```python
from build123d import *

# Parameters (mm, degrees)
STOCK_BOX_1_OUTLINE_W   = 122
STOCK_BOX_1_OUTLINE_H   = 102
STOCK_BOX_1_OUTLINE_W_2 = 118
STOCK_BOX_1_OUTLINE_H_2 = 98
STOCK_BOX_1_DEPTH       = 67
STOCK_BOX_1_2_OUTLINE_W = 118
STOCK_BOX_1_2_OUTLINE_H = 98
STOCK_BOX_1_2_DEPTH     = 2
SKETCH1_W               = 97
SKETCH1_H               = 39.5
CUT_EXTRUDE1_DEPTH      = 10
SKETCH2_W               = 15
SKETCH2_H               = 7.5
CUT_EXTRUDE2_DEPTH      = 10
SKETCH3_W               = 122
SKETCH3_H               = 5
BOSS_EXTRUDE1_DEPTH     = 11
SKETCH5_W               = 122
SKETCH5_H               = 5
BOSS_EXTRUDE2_DEPTH     = 49.5
SKETCH6_W               = 19
SKETCH6_H               = 15
SKETCH6_W_2             = 11
SKETCH6_H_2             = 11
CUT_EXTRUDE3_DEPTH      = 50


# Read off the part's stored shape, not the designer's step: Stock-Box-1
with BuildPart() as part:
    # Stock-Box-1 outline → Stock-Box-1 (new body)
    with BuildSketch(Plane(origin=(0, 0, 0), x_dir=(1, 0, 0), z_dir=(0, 1, 0))):
        with Locations((6.476673428, -22.886409736)):
            Rectangle(STOCK_BOX_1_OUTLINE_W, STOCK_BOX_1_OUTLINE_H)
        with Locations((6.476673428, -22.886409736)):
            Rectangle(STOCK_BOX_1_OUTLINE_W_2, STOCK_BOX_1_OUTLINE_H_2, mode=Mode.SUBTRACT)
    extrude(amount=STOCK_BOX_1_DEPTH)

    # Stock-Box-1 2 outline → Stock-Box-1 2 (add)
    with BuildSketch(Plane(origin=(0, 0, 0), x_dir=(1, 0, 0), z_dir=(0, 1, 0))):
        with Locations((6.476673428, -22.886409736)):
            Rectangle(STOCK_BOX_1_2_OUTLINE_W, STOCK_BOX_1_2_OUTLINE_H)
    extrude(amount=STOCK_BOX_1_2_DEPTH)

    # Sketch1 → Cut-Extrude1 (cut)
    with BuildSketch(Plane.XY.offset(73.886409736)):
        with Locations((6.476673428, 34.25)):
            Rectangle(SKETCH1_W, SKETCH1_H)
    extrude(amount=-CUT_EXTRUDE1_DEPTH, mode=Mode.SUBTRACT)

    # Sketch2 → Cut-Extrude2 (cut)
    with BuildSketch(Plane(origin=(0, 0, -28.113590264), x_dir=(-1, 0, 0), z_dir=(0, 0, -1))):
        with Locations((-22.476673428, 58.25)):
            Rectangle(SKETCH2_W, SKETCH2_H)
        with Locations((29.523326572, 58.25)):
            Rectangle(SKETCH2_W, SKETCH2_H)
    extrude(amount=-CUT_EXTRUDE2_DEPTH, mode=Mode.SUBTRACT)

    # Sketch3 → Boss-Extrude1 (add)
    with BuildSketch(Plane(origin=(0, 0, -28.113590264), x_dir=(-1, 0, 0), z_dir=(0, 0, -1))):
        with Locations((-6.476673428, 52)):
            Rectangle(SKETCH3_W, SKETCH3_H)
    extrude(amount=BOSS_EXTRUDE1_DEPTH)

    # Sketch5 → Boss-Extrude2 (add)
    with BuildSketch(Plane.XZ.offset(-49.5)):
        with Locations((6.476673428, -36.613590264)):
            Rectangle(SKETCH5_W, SKETCH5_H)
    extrude(amount=BOSS_EXTRUDE2_DEPTH)

    # Sketch6 → Cut-Extrude3 (cut)
    with BuildSketch(Plane.ZY.offset(54.523326572)):
        with Locations((-3.613590264, 59.5)):
            Rectangle(SKETCH6_W, SKETCH6_H)
        with Locations((21.386409736, 61.5)):
            Rectangle(SKETCH6_W_2, SKETCH6_H_2)
    extrude(amount=-CUT_EXTRUDE3_DEPTH, mode=Mode.SUBTRACT)


solid = part.part
```
Can you work these out from the model? Positions are in its coordinate system, mm. A direction names the side the tool comes from. Give positions to 0.01 mm unless a question says otherwise; leave off trailing zeros. Order: outer loops, then holes, each group sorted by start corner. A loop starts at its lowest first (then second) coordinate and runs counter-clockwise, first axis right, second up. Notation, with made-up numbers: M 63.25,-12 L 88.25,-12 A32 cw 88.25,27 Z; hole C 11,28.5 d2. An arc over 180 degrees is marked long. Write item = value, one per line. Start each with the question number.
Q1. Will these pins go through, and if not, where does the flat tip stop? pin 1 Ø1 at (x, y) = (-53.5, 61) entering from -Z; pin 2 Ø2 at (x, y) = (-29.5, 57.5) entering from -Z; pin 3 Ø10 at (x, z) = (26, 31) entering from -Y; pin 4 Ø4 at (x, z) = (25.5, -36) entering from +Y.
Q2. We'd pull the mould along X, two halves only. Please class faces 1 (the flat face through (6, 0, 22)), 2 (the flat face through (65.477, 34, 24)), 3 (the flat face through (-54.523, 34, 29)): pulls with the +X half, pulls with the -X half, needs draft (parallel to the pull), parting line crosses it, or undercut.
Q3. Suppose I cut it at D-D (z = 51.5). Write out the boundary of the cut face in (x, y).
Q4. Suppose I cut it at B-B (x = -11.5). Write out the boundary of the cut face in (y, z).
Q5. For faces 4 (the flat face through (6, 12, 71.886)), 5 (the flat face through (67.477, 34, 17)), 6 (the flat face through (6, 25, -34.114)), 7 (the flat face through (6, 61, -28.114)), which set-ups out of +Z, -Z, +X, -X, +Y, -Y let a thin tool reach every point of the face, with its end or its side?
Q6. Suppose I cut it at A-A (x = -31.5). Write out the boundary of the cut face in (y, z), plus the area to 4 significant figures.
Q7. I need wall thicknesses on probe 1 along X at (y, z) = (28.5, 24); probe 2 along Z at (x, y) = (10.5, 16); probe 3 along Z at (x, y) = (-2, 60). Which ranges of each line are inside material? Lowest first, please. Write a range as [from, to].
Q8. Suppose I cut it at C-C (y = 37.5). Write out the boundary of the cut face in (x, z), plus the area to 3 significant figures.
Check result:
q1.pin_1 = -28.11
q1.pin_2 = 71.89
q1.pin_3 = 0
q1.pin_4 = 54.5
q2.face_1 = needs draft
q2.face_2 = undercut
q2.face_3 = pulls with the -X half
q3.outline = M -54.52,0 L 67.48,0 L 67.48,67 L 65.48,67 L 65.48,2 L -52.52,2 L -52.52,67 L -54.52,67 Z
q4.outline = M 0,-39.11 L 54.5,-39.11 L 54.5,-28.11 L 67,-28.11 L 67,-26.11 L 2,-26.11 L 2,71.89 L 14.5,71.89 L 14.5,73.89 L 0,73.89 L 0,-28.11 L 49.5,-28.11 L 49.5,-34.11 L 0,-34.11 Z; M 54,71.89 L 67,71.89 L 67,73.89 L 54,73.89 Z
q5.face_4 = +Y
q5.face_5 = +Z, -Z, +X, +Y, -Y
q5.face_6 = +X, -X, -Y
q5.face_7 = -Z, +X, -X, +Y
q6.outline = M 0,-39.11 L 54.5,-39.11 L 54.5,-26.11 L 2,-26.11 L 2,71.89 L 14.5,71.89 L 14.5,73.89 L 0,73.89 L 0,-28.11 L 49.5,-28.11 L 49.5,-34.11 L 0,-34.11 Z; M 54,71.89 L 67,71.89 L 67,73.89 L 54,73.89 Z; M 62,-28.11 L 67,-28.11 L 67,-26.11 L 62,-26.11 Z
q6.area = 672.5 mm2
q7.probe_1 = [-54.52, -52.52], [65.48, 67.48]
q7.probe_2 = [-39.11, -34.11], [-28.11, -26.11]
q7.probe_3 = [-28.11, -26.11], [71.89, 73.89]
q8.outline = M -54.52,-39.11 L 67.48,-39.11 L 67.48,-34.11 L -54.52,-34.11 Z; M -54.52,-28.11 L 67.48,-28.11 L 67.48,73.89 L 54.98,73.89 L 54.98,71.89 L 65.48,71.89 L 65.48,-26.11 L -52.52,-26.11 L -52.52,71.89 L -42.02,71.89 L -42.02,73.89 L -54.52,73.89 Z
q8.area = 1,300 mm2
